For this review, take the finished solid that the model builds, in its own axes (mm). A direction names the side the tool comes from. Round coordinates to 2 decimals unless told otherwise and drop trailing zeros. Loops run counter-clockwise (first coordinate to the right, second up) from the corner with the lowest first, then second, coordinate; pieces in that order, holes last. Notation, with made-up numbers: (-7, -28) -> (15, -28) arc R13 ccw to (15, -10) -> close; hole circle Ø11 at (-15.75, 65.25). An arc over 180 degrees is marked (long way). Write each question's results on one line, items separated by ' | '.
```python
from build123d import *

# Parameters (mm, degrees)
SKETCH1_W                = 250
SKETCH1_H                = 150
BOSS_EXTRUDE1_DEPTH      = 30
SKETCH2_W                = 230
SKETCH2_H                = 130
CUT_EXTRUDE1_DEPTH       = 20
FILLET1_R                = 10
SKETCH3_W                = 9.75
SKETCH3_H                = 14.5
BOSS_EXTRUDE2_DEPTH      = 10
BOSS_EXTRUDE2_DEPTH_BACK = 10
FILLET3_R                = 2.5
SKETCH4_W                = 250.5
SKETCH4_H                = 135.53043316
CUT_EXTRUDE3_DEPTH       = 36
SKETCH5_W                = 10
SKETCH5_H                = 35
SKETCH5_R                = 1.25
BOSS_EXTRUDE5_DEPTH      = 4
FILLET4_R                = 2.5


with BuildPart() as part:
    # Sketch1 → Boss-Extrude1 (new body)
    with BuildSketch(Plane(origin=(0, 0, 0), x_dir=(1, 0, 0), z_dir=(0, 1, 0))):
        Rectangle(SKETCH1_W, SKETCH1_H)
    extrude(amount=BOSS_EXTRUDE1_DEPTH)

    # Sketch2 → Cut-Extrude1 (cut)
    with BuildSketch(Plane(origin=(0, 30, 0), x_dir=(1, 0, 0), z_dir=(0, 1, 0))):
        Rectangle(SKETCH2_W, SKETCH2_H)
    extrude(amount=-CUT_EXTRUDE1_DEPTH, mode=Mode.SUBTRACT)

    # Fillet1
    fillet1_edges = [part.edges().sort_by_distance(p)[0] for p in [
        (0, 0, 75),
        (-125, 0, 0),
        (0, 0, -75),
        (125, 0, 0),
        (125, 15, 75),
        (-125, 15, 75),
        (-125, 15, -75),
        (125, 15, -75),
    ]]
    fillet(fillet1_edges, radius=FILLET1_R)

    # Sketch3 → Boss-Extrude2 (add, two sides)
    with BuildSketch(Plane(origin=(0, 30, 0), x_dir=(1, 0, 0), z_dir=(0, 1, 0))) as boss_extrude2_sk:
        with Locations((-129.875, 50)):
            Rectangle(SKETCH3_W, SKETCH3_H)
        with Locations((-129.875, -50)):
            Rectangle(SKETCH3_W, SKETCH3_H)
        with Locations((129.875, -50)):
            Rectangle(SKETCH3_W, SKETCH3_H)
        with Locations((129.875, 50)):
            Rectangle(SKETCH3_W, SKETCH3_H)
    extrude(amount=BOSS_EXTRUDE2_DEPTH)
    extrude(boss_extrude2_sk.sketch, amount=-BOSS_EXTRUDE2_DEPTH_BACK)

    # Fillet3
    fillet3_edges = [part.edges().sort_by_distance(p)[0] for p in [
        (125, 20, -50),
        (125, 25, -42.75),
        (125, 25, -57.25),
        (129.875, 20, -57.25),
        (134.75, 20, -50),
        (129.875, 20, -42.75),
        (-125, 20, -50),
        (-125, 25, -57.25),
        (-125, 25, -42.75),
        (-129.875, 20, -42.75),
        (-134.75, 20, -50),
        (-129.875, 20, -57.25),
        (-125, 20, 50),
        (-125, 25, 42.75),
        (-125, 25, 57.25),
        (-129.875, 20, 57.25),
        (-134.75, 20, 50),
        (-129.875, 20, 42.75),
        (125, 20, 50),
        (125, 25, 57.25),
        (125, 25, 42.75),
        (129.875, 20, 42.75),
        (134.75, 20, 50),
        (129.875, 20, 57.25),
    ]]
    fillet(fillet3_edges, radius=FILLET3_R)

    # Sketch4 → Cut-Extrude3 (cut)
    with BuildSketch(Plane(origin=(0, 30, 0), x_dir=(1, 0, 0), z_dir=(0, 1, 0))):
        Rectangle(SKETCH4_W, SKETCH4_H)
    extrude(amount=CUT_EXTRUDE3_DEPTH, mode=Mode.SUBTRACT)

    # Sketch5 → Boss-Extrude5 (add)
    with BuildSketch(Plane(origin=(0, 30, 0), x_dir=(1, 0, 0), z_dir=(0, 1, 0))):
        with Locations((-130, 0)):
            Rectangle(SKETCH5_W, SKETCH5_H)
        with Locations((-130, 10)):
            Circle(SKETCH5_R, mode=Mode.SUBTRACT)
        with Locations((-130, -10)):
            Circle(SKETCH5_R, mode=Mode.SUBTRACT)
    extrude(amount=-BOSS_EXTRUDE5_DEPTH)

    # Fillet4
    fillet4_edges = [part.edges().sort_by_distance(p)[0] for p in [
        (-125, 28, -17.5),
        (-125, 28, 17.5),
        (-135, 28, 17.5),
        (-135, 28, -17.5),
    ]]
    fillet(fillet4_edges, radius=FILLET4_R)


solid = part.part
```
1. Tool access review of faces 1 (the face through (-130, 31, 42.75)), 2 (the face through (-2, 20, 65)), 3 (the face through (125.25, 35, -50)): name each direction out of +Z, -Z, +X, -X, +Y, -Y from which nothing blocks a thin tool from reaching the whole face with its end or side.
Values found:
face 1: -X, +Y | face 2: +Y | face 3: +Z, -Z, +Y
2. For pin 1 (4 mm diameter, centred on x = 77.5, y = 6.5, fed in from +Z); pin 2 (10.5 mm diameter, centred on x = -131.5, y = 31, fed in from +Z); pin 3 (10 mm diameter, centred on y = 20.5, z = -12.5, fed in from -X), all flat-tipped, find the tip position at first contact; note any pin that passes through.
Values found:
pin 1: stops at z = 74.89 | pin 2: stops at z = 57.53 | pin 3: stops at x = -125
3. Consider section C-C (z = 22.5). State the section outline as (x, y) points, plus the area to 3 significant figures.
Values found:
outline: (-125, 10) arc R10 ccw to (-115, 0) -> (115, 0) arc R10 ccw to (125, 10) -> (125, 30) -> (115, 30) -> (115, 10) -> (-115, 10) -> (-115, 30) -> (-125, 30) -> close | area: 2,860 mm2
4. Consider section B-B (z = -48.5). State the section outline as (x, y) points, plus the area to 3 significant figures.
Values found:
outline: (-134.75, 22.5) arc R2.5 ccw to (-132.25, 20) -> (-127.5, 20) arc R2.5 cw to (-125, 17.5) -> (-125, 10) arc R10 ccw to (-115, 0) -> (115, 0) arc R10 ccw to (125, 10) -> (125, 17.5) arc R2.5 cw to (127.5, 20) -> (132.25, 20) arc R2.5 ccw to (134.75, 22.5) -> (134.75, 40) -> (125.25, 40) -> (125.25, 30) -> (115, 30) -> (115, 10) -> (-115, 10) -> (-115, 30) -> (-125.25, 30) -> (-125.25, 40) -> (-134.75, 40) -> close | area: 3,240 mm2
5. To check wall thickness, follow probe 1 along X at (y, z) = (28.6, 10); probe 2 along Z at (x, y) = (-130, 28); probe 3 along X at (y, z) = (24.5, 54). State the ranges of each line that lie inside material, in increasing order.
Values found:
probe 1: x = -135 to -131.25, -128.75 to -115, 115 to 125 | probe 2: z = -57.25 to -42.75, -17.5 to -11.25, -8.75 to 8.75, 11.25 to 17.5, 42.75 to 57.25 | probe 3: x = -134.75 to -115, 115 to 134.75
6. Consider section A-A (x = -27). State the section outline as (y, z) points.
Values found:
outline: (0, -65) arc R10 ccw to (10, -75) -> (30, -75) -> (30, -65) -> (10, -65) -> (10, 65) -> (30, 65) -> (30, 75) -> (10, 75) arc R10 ccw to (0, 65) -> close
7. Draft analysis for pull direction X (two halves, no side actions). For faces 4 (the face through (-2, 10, -1)), 5 (the face through (-122.15, 3.01, -0.91)), 6 (the face through (130, 20, 50)), state which applies: released by +X, released by -X, zero draft, split by the parting line, or undercut.
Values found:
face 4: undercut | face 5: released by -X | face 6: zero draft
